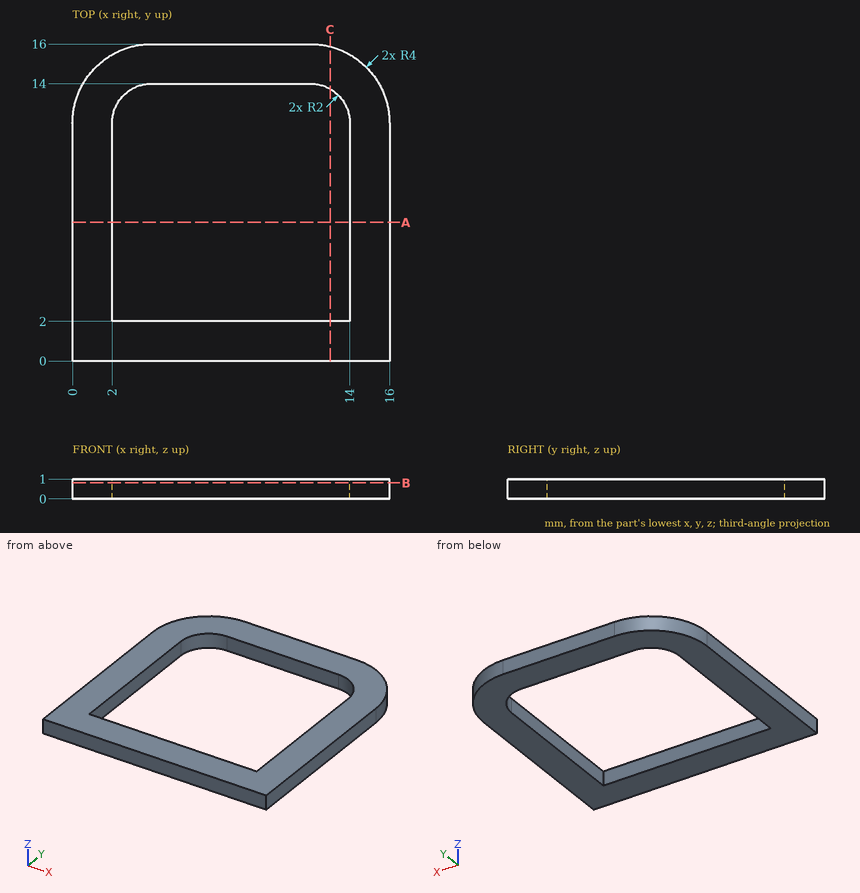
Can you work these out from the drawing? Everything is in mm from the part's minimum corner. Round coordinates to 2 decimals unless told otherwise and drop trailing zeros. Order: outer loops, then holes, each group sorted by start corner. A loop starts at its lowest first (then second) coordinate and runs counter-clockwise, first axis right, second up. Notation, with made-up numbers: (4, 78.5) -> (50, 78.5) arc R20 cw to (50, 112.5) -> close; hole circle Ø10 at (-5, 45.25). An arc over 180 degrees is marked (long way). Return JSON: item names as keys, results as strings. Group by question number.
1. I need wall thicknesses on line 1 (X direction, y = 6.5, z = 0.55); line 2 (Y direction, x = 12.5, z = 0.7). Which ranges of each line are inside material? Lowest first, please. Write a range as [from, to].
2. If we section it at B-B, the plane z = 0.8: Write out the boundary of the cut face in (x, y), then the cut area to 3 significant figures.
3. If we section it at C-C, the plane x = 13: Write out the boundary of the cut face in (y, z).
4. If we section it at A-A, the plane y = 7: Write out the boundary of the cut face in (x, z), then the cut area to 3 significant figures.
Output values:
{
 "1": {"line 1": "[0, 2], [14, 16]", "line 2": "[0, 2], [13.94, 15.97]"},
 "2": {"outline": "(0, 0) -> (16, 0) -> (16, 12) arc R4 ccw to (12, 16) -> (4, 16) arc R4 ccw to (0, 12) -> close; hole (2, 2) -> (14, 2) -> (14, 12) arc R2 ccw to (12, 14) -> (4, 14) arc R2 ccw to (2, 12) -> close", "area": "107 mm²"},
 "3": {"outline": "(0, 0) -> (2, 0) -> (2, 1) -> (0, 1) -> close; (13.73, 0) -> (15.87, 0) -> (15.87, 1) -> (13.73, 1) -> close"},
 "4": {"outline": "(0, 0) -> (2, 0) -> (2, 1) -> (0, 1) -> close; (14, 0) -> (16, 0) -> (16, 1) -> (14, 1) -> close", "area": "4.00 mm²"}
}
